Read the model definition and answer for the solid it produces. Units are mm, in the model's axes. A direction names the side the tool comes from. Round coordinates to 2 decimals unless told otherwise and drop trailing zeros. Loops run counter-clockwise (first coordinate to the right, second up) from the corner with the lowest first, then second, coordinate; pieces in that order, holes last. Notation, with made-up numbers: (68, 29) - (99, 29) arc R18 cw to (99, 44) - close; hole circle Ø8 at (89.5, -28). An arc over 180 degrees is marked (long way). Answer as CSV lines item,"result".
```python
from build123d import *

# Parameters (mm, degrees)
F1_DEPTH = 6.35
F2_R     = 9.525
F3_DEPTH = 25.4
F5_SCALE = 0.5


with BuildPart() as f1:
    # F0 (on Front) → F1 (new body)
    with BuildSketch(Plane.XZ):
        Polygon((7.211127909, -9.756404553), (9.8366258623, 5.8999802627), (-2.4094521428, 16.0019205958), (-17.2810281013, 10.4474761131), (-19.9065260547, -5.2089087026), (-7.6604480495, -15.3108490356), align=None)
    extrude(amount=F1_DEPTH)

    # F2 (on face) → F3 (join)
    with BuildSketch(Plane.XZ.offset(6.35)):
        with Locations((-5.0349500962, 0.3455357801)):
            Circle(F2_R)
    extrude(amount=F3_DEPTH)

    # F4: F1 across face


with BuildPart() as f1_1:
    add(f1.part)
    add(f1.part.mirror(Plane(origin=(-5.0349500962, 0, 0.3455357801), x_dir=(1, 0, 0), z_dir=(0, 1, 0))))


with BuildPart() as f1_2:
    # F5: moved
    add(f1_1.part.scale(F5_SCALE))


solid = f1_2.part
```
1) A cutting plane is placed at D-D, the plane z = -6. Determine the outline of the cut face in (x, y) (3 decimals).
Entries:
outline,"(-5.837, -3.175) - (0.602, -3.175) - (0.602, 3.175) - (-5.837, 3.175) - close"
2) Find the intervals of material crossed by line 1 (Y direction, x = -7.5, z = 0.5) (3 decimals); line 2 (Z direction, x = -2.75, y = 4); line 3 (X direction, y = -8.5, z = 0.25), in increasing order.
Entries:
line 1,"y = -3.175 to 3.175"
line 2,"z = -4.58 to 4.93"
line 3,"x = -7.28 to 2.24"
3) Each of these flat-tipped pins is pushed along its axis until it touches: P1, Ø1.5, axis at y = 5.5, z = 4.5, coming from the -X side; P2, Ø5, axis at x = 2.5, y = -2, coming from the +Z side; P3, Ø6, axis at y = -3.5, z = 4.5, coming from the +X side; P4, Ø2, axis at y = -0.5, z = 3.5, coming from the -X side. Where does it stop, or does it pass through?
Entries:
P1,"stops at x = -5.66"
P2,"stops at z = 7.01"
P3,"stops at x = 4.92"
P4,"stops at x = -9.1"
4) A tool of negligible diameter and unlimited length cuts with its end or side. For faces 1 (the face through (-6.935, -0.044, -5.095)), 2 (the face through (-6, 3.175, 4)), 3 (the face through (-6, -3.175, 4)), from which of +Z, -Z, +X, -X, +Y, -Y can it reach the whole face along a straight path? Write none if from no direction.
Entries:
face 1,"-Z, -X, +Y, -Y"
face 2,"+Y"
face 3,"-Y"
5) A cutting plane is placed at A-A, the plane x = -4.5. Determine the outline of the cut face in (y, z) (3 decimals).
Entries:
outline,"(-15.875, -4.157) - (-3.175, -4.157) - (-3.175, -7.103) - (3.175, -7.103) - (3.175, -4.157) - (15.875, -4.157) - (15.875, 4.503) - (3.175, 4.503) - (3.175, 6.77) - (-3.175, 6.77) - (-3.175, 4.503) - (-15.875, 4.503) - close"
6) A cutting plane is placed at B-B, the plane z = -0.75. Determine the outline of the cut face in (x, y) (3 decimals).
Entries:
outline,"(-9.642, -3.175) - (-7.19, -3.175) - (-7.19, -15.875) - (2.155, -15.875) - (2.155, -3.175) - (4.298, -3.175) - (4.298, 3.175) - (2.155, 3.175) - (2.155, 15.875) - (-7.19, 15.875) - (-7.19, 3.175) - (-9.642, 3.175) - close"
7) A cutting plane is placed at C-C, the plane y = -12. Determine the outline of the cut face in (x, z) (1 decimal).
Entries:
outline,"circle Ø9.5 at (-2.5, 0.2)"
